The listing builds one solid part. Answer for the finished solid, in the listing's coordinates (mm). A direction names the side the tool comes from. Round coordinates to 2 decimals unless told otherwise and drop trailing zeros. Order: outer loops, then holes, each group sorted by start corner. A loop starts at its lowest first (then second) coordinate and runs counter-clockwise, first axis right, second up. Notation, with made-up numbers: M -36.75,65 L -10.75,65 A18 cw -10.75,99 Z; hole C -26.75,-14 d6. An arc over 180 degrees is marked long. Write item = value, one per line. Start each with the question number.
(1) A cutting plane is placed at B-B, the plane y = 7.25. Determine the outline of the cut face in (x, z) (3 decimals), and give its area (3 significant figures).
(2) Straight lines are drawn through the part: probe 1 along X at (y, z) = (0.6, -1.46); probe 2 along Z at (x, y) = (-6.54, 1.1); probe 3 along X at (y, z) = (1, -46.5). For each, find the intervals that lie inside material, in ascending order. Write a range as from..to.
(3) A cutting plane is placed at D-D, the plane z = -10.5. Determine the outline of the cut face in (x, y), and give its area (3 significant figures).
(4) Each of these flat-tipped pins is pushed along its axis until it touches: pin 1 (5 mm diameter, centred on x = 19.5, z = -2, fed in from -Y); pin 2 (2 mm diameter, centred on y = 10.5, z = -28, fed in from -X); pin 3 (2.5 mm diameter, centred on x = 39, z = -83.5, fed in from -Y); pin 4 (1.6 mm diameter, centred on x = -5, y = 1.5, fed in from -Z). Where does it stop, or does it pass through?
(5) For a pull along Z with two mould halves and no side action, classify faces 1 (the face through (27, 6, 2.54)), 2 (the face through (-6, 2, -30)), 3 (the face through (28, 5, 0)) as released by +Z, released by -Z, zero draft, split by the parting line, or undercut.
(6) A cutting plane is placed at C-C, the plane x = 43. Determine the outline of the cut face in (y, z) (1 decimal).
(7) Which of the six approach directions +Z, -Z, +X, -X, +Y, -Y give full straight-line access (tool end or side, diameter ignored) to faces 4 (the face through (29, 5, -85.725)), 5 (the face through (-7, 1.01, -54.91)), 6 (the face through (-5, 1, -60.96))?
(8) A cutting plane is placed at A-A, the plane z = -66.5. Determine the outline of the cut face in (x, y), and give its area (3 significant figures).
Autodesk Inventor part; units mm, degrees
ref_plane "YZ Plane" through (0, 0, 0) normal (1, 0, 0) x (0, 1, 0)
ref_plane "XZ Plane" through (0, 0, 0) normal (0, 1, 0) x (-1, 0, 0)
ref_plane "XY Plane" through (0, 0, 0) normal (0, 0, 1) x (1, 0, 0)
sketch "Sketch1" plane through (0, 0, 0) normal (0, 1, 0) x (-1, 0, 0)
  line L0 (0, 0) -> (-57.15, 0)
  line L1 (-57.15, 0) -> (-57.15, -85.725)
  line L2 (-57.15, -85.725) -> (0, -85.725)
  line L3 (0, -85.725) -> (0, 0)
  line L4 (-59.69, -88.265) -> (-59.69, 2.54)
  line L5 (-59.69, 2.54) -> (2.54, 2.54)
  line L6 (2.54, 2.54) -> (2.54, -88.265)
  line L7 (2.54, -88.265) -> (-59.69, -88.265)
  dimension "d0" = 57.15
  dimension "d1" = 85.725
  dimension "d2" = 2.54
extrude "Extrusion1" add sketch "Sketch1" along normal blind 11.1125
sketch "Sketch2" plane through (0, 11.1125, 0) normal (0, 1, 0) x (1, 0, 0)
  line L0 (57.15, 0) -> (0, 0)
  line L1 (0, 85.725) -> (57.15, 85.725)
  line L2 (0, 0) -> (0, 85.725)
  line L3 (57.15, 85.725) -> (57.15, 0)
  line L4 (0, 85.725) -> (57.15, 85.725)
  line L5 (57.15, 85.725) -> (57.15, 80.9625)
  line L6 (57.15, 80.9625) -> (0, 80.9625)
  line L7 (0, 80.9625) -> (0, 85.725)
  line L8 (59.69, 88.265) -> (-2.54, 88.265)
  line L9 (-2.54, -2.54) -> (59.69, -2.54)
  line L10 (0, 0) -> (57.15, 0)
  line L11 (57.15, 0) -> (57.15, 4.7625)
  line L12 (57.15, 4.7625) -> (0, 4.7625)
  line L13 (0, 4.7625) -> (0, 0)
  line L14 (0, 0) -> (0, 85.725)
  line L15 (0, 85.725) -> (57.15, 85.725)
  line L16 (57.15, 85.725) -> (57.15, 0)
  line L17 (57.15, 0) -> (0, 0)
  line L18 (59.69, -2.54) -> (59.69, 88.265)
  line L19 (59.69, 88.265) -> (-2.54, 88.265)
  line L20 (-2.54, 88.265) -> (-2.54, -2.54)
  line L21 (-2.54, -2.54) -> (59.69, -2.54)
  dimension "d5" = 4.7625
  dimension "d6" = 4.7625
extrude "Extrusion2" add sketch "Sketch2" along normal blind 1.5875 contours L0 L2 L12 L3 | L6 L2 L1 L3 | L18 L9 L20 L8
sketch "Sketch4" plane through (-2.54, 0, -88.265) normal (-1, 0, 0) x (0, 0, 1)
  line L0 (90.805, 0) -> (0, 0)
  line L1 (90.805, 0) -> (90.805, 12.7)
  line L2 (0, 12.7) -> (90.805, 12.7)
  line L3 (0, 0) -> (0, 12.7)
  line L4 (90.805, 0) -> (90.805, 12.7)
  line L5 (90.805, 0) -> (27.305, 0)
  line L6 (27.305, 0) -> (27.305, 2)
  line L7 (27.305, 2) -> (90.805, 2)
  line L8 (90.805, 2) -> (90.805, 0)
  point P0 (88.265, 0)
  dimension "d13" = 63.5
  dimension "d14" = 2
extrude "Extrusion4" add sketch "Sketch4" along normal blind 8 contours L0 L6 L7 L1
fillet "Fillet2" radius 4 2 edges at (-10.54, 1, 2.54) (-10.54, 1, -60.96)
sketch "Sketch5" plane through (-2.54, 2, 2.54) normal (0, 1, 0) x (1, 0, 0)
  line L0 (-8, 4) -> (-8, 59.5)
  line L1 (-8, 4) -> (0, 4)
  line L2 (0, 63.5) -> (0, 0)
  circle A0 centre (-4, 4) radius 2.1
  line L3 (-8, 59.5) -> (0, 59.5)
  circle A1 centre (-4, 59.5) radius 2.1
  point P0 (2.54, 2.54)
  dimension "d20" = 4.2
  dimension "d21" = 4.2
extrude "Extrusion5" cut sketch "Sketch5" against normal up to next contours A0 L1 | L1 A0 | A1 L3 | L3 A1
properties part number "MiniBreadboardHolder"
Reported:
q1.outline = M -2.54,-88.265 L 59.69,-88.265 L 59.69,2.54 L -2.54,2.54 Z; hole M 0,-85.725 L 57.15,-85.725 L 57.15,0 L 0,0 Z
q1.area = 752 mm²
q2.probe_1 = -10.54..-8.64, -4.44..0, 57.15..59.69
q2.probe_2 = -60.96..-59.06, -54.86..-3.56, 0.64..2.54
q2.probe_3 = -10.54..0, 57.15..59.69
q3.outline = M -10.54,0 L 0,0 L 0,12.7 L -2.54,12.7 L -2.54,2 L -10.54,2 Z; M 57.15,0 L 59.69,0 L 59.69,12.7 L 57.15,12.7 Z
q3.area = 80.5 mm²
q4.pin_1 = 0
q4.pin_2 = -2.54
q4.pin_3 = 11.11
q4.pin_4 = -60.96
q5.face_1 = released by +Z
q5.face_2 = zero draft
q5.face_3 = undercut
q6.outline = M 0,-88.3 L 12.7,-88.3 L 12.7,-81 L 11.1,-81 L 11.1,-85.7 L 0,-85.7 Z; M 0,0 L 11.1,0 L 11.1,-4.8 L 12.7,-4.8 L 12.7,2.5 L 0,2.5 Z
q7.face_4 = -Y
q7.face_5 = +Y, -Y
q7.face_6 = -Z, -X, +Y, -Y
q8.outline = M -2.54,0 L 0,0 L 0,12.7 L -2.54,12.7 Z; M 57.15,0 L 59.69,0 L 59.69,12.7 L 57.15,12.7 Z
q8.area = 64.5 mm²
